For this review, take the finished solid that the model builds, in its own axes (mm). A direction names the side the tool comes from. Give positions to 0.01 mm unless a question says otherwise; leave off trailing zeros. Write each loop counter-clockwise with the first axis right and the second up, starting at its lowest first coordinate (ties: lowest second). Pieces come first, ordered by that corner, then holes.
1) We need section C-C on y = 0. Give the boundary of the cut face in (x, z), and give its area (3 significant figures).
2) We need section A-A on x = 0. Give the boundary of the cut face in (y, z) (3 decimals), and give its area (3 significant figures).
3) We need section D-D on z = -26. Give the boundary of the cut face in (x, y), and give its area (3 significant figures).
4) For P1, Ø2, axis at x = 2, z = -27.5, coming from the +Y side; P2, Ø3, axis at x = 2, y = -2, coming from the -Z side; P3, Ø2, axis at y = -1, z = -47.5, coming from the -X side; P4, Ø1.2, axis at y = 0, z = -49.5, coming from the +X side, all flat-tipped, find the tip position at first contact; note any pin that passes through.
5) Machinability: for faces 5 (the face through (0, -2.7, -49.2)), 6 (the face through (-1.8, 0, -49)), 7 (the face through (2, 0, -45.5)), 8 (the face through (1.8, 0, -49)), 9 (the face through (0.028, 2.725, -2.676)), which of the approach directions +Z, -Z, +X, -X, +Y, -Y give a long, thin tool a straight path to every point of the face, cutting with its end or side? Answer none if there is none.
6) We need section B-B on z = -0.5. Give the boundary of the cut face in (x, y) (3 decimals).
7) Wall thickness on line 1 along Z through (x, y) = (2.25, -0.75); line 2 along X through (y, z) = (3, -43); line 3 along Z through (x, y) = (-1, 1.5): over which ranges is each line inside the solid? List them lowest first.
8) Draft analysis for pull direction Y (two halves, no side actions). For faces 1 (the face through (0, 0, -53)), 2 (the face through (-0.028, -2.725, -2.676)), 3 (the face through (0, 2.7, -49.2)), 4 (the face through (3.233, -1.341, -21.164)), state which applies: pulls with the +Y half, pulls with the -Y half, needs draft (parallel to the pull), parting line crosses it, or undercut.
from build123d import *

# Parameters (mm, degrees)
CROQUIS1_R              = 3.5
SALIENTE_EXTRUIR1_DEPTH = 65.5
CORTAR_EXTRUIR3_DEPTH   = 8
CORTAR_EXTRUIR5_START   = -20
CROQUIS7_R              = 3.5
CORTAR_EXTRUIR5_DEPTH   = 20
CROQUIS8_W              = 12.617225576
CROQUIS8_H              = 9.28288649
CORTAR_EXTRUIR6_DEPTH   = 10
SALIENTE_EXTRUIR2_START = 2.5
CROQUIS10_R             = 3.5
SALIENTE_EXTRUIR2_DEPTH = 2.5


with BuildPart() as part:
    # Croquis1 → Saliente-Extruir1 (new body)
    with BuildSketch(Plane.XY):
        Circle(CROQUIS1_R)
    extrude(amount=-SALIENTE_EXTRUIR1_DEPTH)

    # Croquis6 → Cortar-Extruir3 (cut)
    with BuildSketch(Plane.XY):
        with BuildLine():
            Line((-1.8, 2.045880006), (-1.8, -2.045880006))
            ThreePointArc((-1.8, -2.045880006), (0, -2.725), (1.8, -2.045880006))
            Line((1.8, -2.045880006), (1.8, 2.045880006))
            ThreePointArc((1.8, 2.045880006), (0, 2.725), (-1.8, 2.045880006))
        make_face()
    extrude(amount=-CORTAR_EXTRUIR3_DEPTH, mode=Mode.SUBTRACT)

    # Croquis7 → Cortar-Extruir5 (cut)
    with BuildSketch(Plane(origin=(0, 0, -65.5), x_dir=(-1, 0, 0), z_dir=(0, 0, -1)).offset(CORTAR_EXTRUIR5_START)):
        with Locations(Location((0, 0, 0), (0, 0, 180))):
            Circle(CROQUIS7_R)
        with BuildLine():
            ThreePointArc((1.8, 2.01246118), (0, 2.7), (-1.8, 2.01246118))
            Line((-1.8, 2.01246118), (-1.8, -2.01246118))
            ThreePointArc((-1.8, -2.01246118), (0, -2.7), (1.8, -2.01246118))
            Line((1.8, -2.01246118), (1.8, 2.01246118))
        make_face(mode=Mode.SUBTRACT)
    extrude(amount=CORTAR_EXTRUIR5_DEPTH, mode=Mode.SUBTRACT)

    # Croquis8 → Cortar-Extruir6 (cut)
    with BuildSketch(Plane.ZY.offset(1.8)):
        with Locations((-59.308612788, -0.436721269)):
            Rectangle(CROQUIS8_W, CROQUIS8_H)
    extrude(amount=-CORTAR_EXTRUIR6_DEPTH, mode=Mode.SUBTRACT)

    # Croquis10 → Saliente-Extruir2 (add)
    with BuildSketch(Plane.XY.offset(SALIENTE_EXTRUIR2_START)):
        Circle(CROQUIS10_R)
        with BuildLine():
            Line((-1.8, 2.045880006), (-1.8, -2.045880006))
            ThreePointArc((-1.8, -2.045880006), (0, -2.725), (1.8, -2.045880006))
            Line((1.8, -2.045880006), (1.8, 2.045880006))
            ThreePointArc((1.8, 2.045880006), (0, 2.725), (-1.8, 2.045880006))
        make_face(mode=Mode.SUBTRACT)
    extrude(amount=-SALIENTE_EXTRUIR2_DEPTH)


solid = part.part
Results list:
1. outline: (-3.5, -45.5) - (-1.8, -45.5) - (-1.8, -53) - (1.8, -53) - (1.8, -45.5) - (3.5, -45.5) - (3.5, 2.5) - (1.8, 2.5) - (1.8, -8) - (-1.8, -8) - (-1.8, 2.5) - (-3.5, 2.5) - close
1. area: 325 mm2
2. outline: (-3.5, -45.5) - (-2.7, -45.5) - (-2.7, -53) - (2.7, -53) - (2.7, -45.5) - (3.5, -45.5) - (3.5, 2.5) - (2.725, 2.5) - (2.725, -8) - (-2.725, -8) - (-2.725, 2.5) - (-3.5, 2.5) - close
2. area: 319 mm2
3. outline: circle Ø7 at (0, 0)
3. area: 38.5 mm2
4. P1: stops at y = 3.35
4. P2: stops at z = -53
4. P3: stops at x = -1.8
4. P4: stops at x = 1.8
5. face 5: -Z, -Y
5. face 6: -Z, -X, +Y, -Y
5. face 7: -Z
5. face 8: -Z, +X, +Y, -Y
5. face 9: +Z
6. outline: circle Ø7 at (0, 0); hole (-1.8, -2.046) arc R2.725 ccw to (1.8, -2.046) - (1.8, 2.046) arc R2.725 ccw to (-1.8, 2.046) - close
7. line 1: z = -45.5 to 2.5
7. line 2: x = -1.8 to 1.8
7. line 3: z = -53 to -8
8. face 1: needs draft
8. face 2: undercut
8. face 3: pulls with the +Y half
8. face 4: parting line crosses it
